Here's how the part is built. I have some questions about the finished solid (model axes, mm). A direction names the side the tool comes from. Round coordinates to 2 decimals unless told otherwise and drop trailing zeros. Write each loop counter-clockwise with the first axis right and the second up, starting at its lowest first coordinate (ties: lowest second). Pieces come first, ordered by that corner, then holes. Notation, with made-up numbers: (27.25, 58.5) -> (52.25, 58.5) arc R34 ccw to (52.25, 93.5) -> close; hole circle Ø11 at (-28, -10.5). An arc over 180 degrees is marked (long way). Put each result on its own line as item: value. Start each with the question number.
1. Suppose I cut it at A-A (z = 25.5). Count the separate pieces of the cut face and the enclosed holes in it, then the cut area to 3 significant figures.
2. For pin 1 (0.9 mm diameter, centred on y = 0.5, z = 17, fed in from -X) (3 decimals); pin 2 (0.9 mm diameter, centred on y = 0.5, z = 16.5, fed in from +X) (3 decimals), each with a flat end and sliding along its axis, tell me the tip position at first contact or that it passes through.
3. I need wall thicknesses on probe 1 along X at (y, z) = (0.5, 27) (3 decimals); probe 2 along Z at (x, y) = (-2, 0.5); probe 3 along X at (y, z) = (1.25, 6.5) (3 decimals). Which ranges of each line are inside material? Lowest first, please. Write a range as from..to.
4. Suppose I cut it at C-C (z = 16.51). Please give me the cut outline in (x, y) (3 decimals), then the cut area to 3 significant figures.
5. We'd pull the mould along Y, two halves only. Please class faces 1 (the face through (0, -6.35, 16)), 2 (the face through (-24.33, 0.07, 15.01)), 3 (the face through (28.275, 2, 16)): +Y half, -Y half, draft (parallel to the pull), parting line (faces both ways), or undercut.
6. Which directions (+Z, -Z, +X, -X, +Y, -Y) give clear straight access to the entire face, cutting with the end or side of a thin tool? Please do faces 4 (the face through (0, 7.144, 16)), 5 (the face through (-24.331, -0.575, 7.736)), 6 (the face through (20.275, 0, 6)), 7 (the face through (-18.96, 0.07, 26.82)).
```python
from build123d import *

# Parameters (mm, degrees)
SKETCH1_W           = 56.55
SKETCH1_H           = 12.7
BOSS_EXTRUDE1_DEPTH = 31.75
SKETCH2_R           = 1.5
SKETCH2_R_2         = 3
CUT_EXTRUDE1_DEPTH  = 10
CUT_EXTRUDE2_DEPTH  = 8
SKETCH4_W           = 56.55
SKETCH4_H           = 31.75
BOSS_EXTRUDE2_DEPTH = 0.79375


with BuildPart() as part:
    # Sketch1 → Boss-Extrude1 (new body)
    with BuildSketch(Plane.XY):
        Rectangle(SKETCH1_W, SKETCH1_H)
    extrude(amount=BOSS_EXTRUDE1_DEPTH)

    # Sketch2 → Cut-Extrude1 (cut)
    with BuildSketch(Plane.XY.offset(31.75)):
        with Locations((-17.4625, 0)):
            Circle(SKETCH2_R)
        Circle(SKETCH2_R_2)
    extrude(amount=-CUT_EXTRUDE1_DEPTH, mode=Mode.SUBTRACT)

    # Sketch3 → Cut-Extrude2 (cut)
    with BuildSketch(Plane.ZY.offset(28.275)):
        with BuildLine():
            ThreePointArc((4.85, 0), (6.35, -1.5), (7.85, 0))
            Line((7.85, 0), (4.85, 0))
        make_face()
        with BuildLine():
            Line((4.85, 0), (7.85, 0))
            ThreePointArc((7.85, 0), (6.35, 1.5), (4.85, 0))
        make_face()
        with BuildLine():
            ThreePointArc((15.01, 0), (16.51, -1.5), (18.01, 0))
            Line((18.01, 0), (15.01, 0))
        make_face()
        with BuildLine():
            Line((15.01, 0), (18.01, 0))
            ThreePointArc((18.01, 0), (16.51, 1.5), (15.01, 0))
        make_face()
    cut_extrude2 = extrude(amount=-CUT_EXTRUDE2_DEPTH, mode=Mode.SUBTRACT)

    # Sketch4 → Boss-Extrude2 (add)
    with BuildSketch(Plane(origin=(0, 6.35, 0), x_dir=(1, 0, 0), z_dir=(0, 1, 0))):
        with Locations((0, -15.875)):
            Rectangle(SKETCH4_W, SKETCH4_H)
    extrude(amount=BOSS_EXTRUDE2_DEPTH)

    # Mirror1: Cut-Extrude2 across plane
    add(cut_extrude2.mirror(Plane(origin=(0, 0, 0), x_dir=(0, 0, 1), z_dir=(1, 0, 0))), mode=Mode.SUBTRACT)


solid = part.part
```
Verdict:
1. separate pieces: 1
1. enclosed holes: 2
1. area: 728 mm^2
2. pin 1: stops at x = -20.275
2. pin 2: stops at x = 20.275
3. probe 1: x = -28.275..-18.877, -16.048..-2.958, 2.958..28.275
3. probe 2: z = 0..21.75
3. probe 3: x = -20.275..20.275
4. outline: (-28.275, -6.35) -> (28.275, -6.35) -> (28.275, -1.5) -> (20.275, -1.5) -> (20.275, 1.5) -> (28.275, 1.5) -> (28.275, 7.144) -> (-28.275, 7.144) -> (-28.275, 1.5) -> (-20.275, 1.5) -> (-20.275, -1.5) -> (-28.275, -1.5) -> close
4. area: 715 mm^2
5. face 1: -Y half
5. face 2: undercut
5. face 3: draft
6. face 4: +Z, -Z, +X, -X, +Y
6. face 5: -X
6. face 6: +X
6. face 7: +Z
